Geometry check sheet. Reference: the model listing, model coordinates, mm. Round coordinates to 2 decimals unless told otherwise and drop trailing zeros. Loops run counter-clockwise (first coordinate to the right, second up) from the corner with the lowest first, then second, coordinate; pieces in that order, holes last. Notation, with made-up numbers: M -19.5,66 L 22.5,66 A25 ccw 22.5,81 Z; hole C 23.25,86.25 d1. An arc over 180 degrees is marked long. Write item = value, one per line.
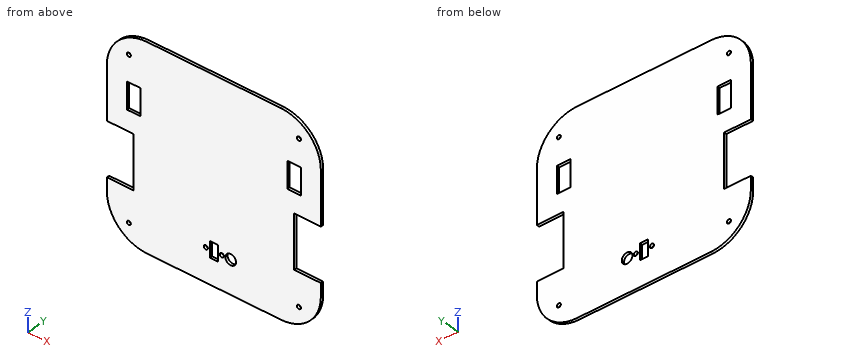
from build123d import *

# Parameters (mm, degrees)
SKETCH1_R           = 1.5
BOSS_EXTRUDE1_DEPTH = 2
SKETCH2_R           = 1.55
SKETCH2_R_2         = 4
SKETCH2_W           = 6
SKETCH2_H           = 12
CUT_EXTRUDE1_DEPTH  = 10
SKETCH3_W           = 10
SKETCH3_H           = 20
CUT_EXTRUDE2_DEPTH  = 10


with BuildPart() as part:
    # Sketch1 → Boss-Extrude1 (new body)
    with BuildSketch(Plane(origin=(0, 0, 0), x_dir=(1, 0, 0), z_dir=(0, 1, 0))):
        with BuildLine():
            Line((-80, 35), (-60, 35))
            Line((-60, 35), (-60, -5))
            Line((-60, -5), (-80, -5))
            Line((-80, -5), (-80, -45))
            ThreePointArc((-80, -45), (-71.213203436, -66.213203436), (-50, -75))
            Line((-50, -75), (50, -75))
            ThreePointArc((50, -75), (71.213203436, -66.213203436), (80, -45))
            Line((80, -45), (80, -5))
            Line((80, -5), (60, -5))
            Line((60, -5), (60, 35))
            Line((60, 35), (80, 35))
            Line((80, 35), (80, 45))
            ThreePointArc((80, 45), (71.213203436, 66.213203436), (50, 75))
            Line((50, 75), (-50, 75))
            ThreePointArc((-50, 75), (-71.213203436, 66.213203436), (-80, 45))
            Line((-80, 45), (-80, 35))
        make_face()
        with Locations(Location((-63.621027185, 59.644712986, 0), (0, 0, 270))):
            Circle(SKETCH1_R, mode=Mode.SUBTRACT)
        with Locations(Location((63.621027185, 59.644712986, 0), (0, 0, 90))):
            Circle(SKETCH1_R, mode=Mode.SUBTRACT)
        with Locations(Location((63.621027185, -59.644712986, 0), (0, 0, 270))):
            Circle(SKETCH1_R, mode=Mode.SUBTRACT)
        with Locations(Location((-63.621027185, -59.644712986, 0), (0, 0, 90))):
            Circle(SKETCH1_R, mode=Mode.SUBTRACT)
    extrude(amount=BOSS_EXTRUDE1_DEPTH)

    # Sketch2 → Cut-Extrude1 (cut)
    with BuildSketch(Plane(origin=(0, 2, 0), x_dir=(1, 0, 0), z_dir=(0, 1, 0))):
        with Locations(Location((-6, 50, 0), (0, 0, 270))):
            Circle(SKETCH2_R)
        with Locations(Location((6, 50, 0), (0, 0, 270))):
            Circle(SKETCH2_R)
        with Locations(Location((12.55, 50, 0), (0, 0, 270))):
            Circle(SKETCH2_R_2)
        with Locations((0, 50)):
            Rectangle(SKETCH2_W, SKETCH2_H)
    extrude(amount=-CUT_EXTRUDE1_DEPTH, mode=Mode.SUBTRACT)

    # Sketch3 → Cut-Extrude2 (cut)
    with BuildSketch(Plane(origin=(0, 2, 0), x_dir=(1, 0, 0), z_dir=(0, 1, 0))):
        with Locations((-60, -30)):
            Rectangle(SKETCH3_W, SKETCH3_H)
        with Locations((60, -30)):
            Rectangle(SKETCH3_W, SKETCH3_H)
    extrude(amount=-CUT_EXTRUDE2_DEPTH, mode=Mode.SUBTRACT)


solid = part.part
(1) Sectioned sample at B-B on z = 2.5. Record the cut outline in (x, y), then the cut area to 3 significant figures.
Result set:
outline = M -60,0 L 60,0 L 60,2 L -60,2 Z
area = 240 mm2
(2) Material ranges on line 1 along Z through (x, y) = (-61, 0.2); line 2 along X through (y, z) = (0.55, -21.5); line 3 along Z through (x, y) = (64.5, 0.9), recorded low to high. Write a range as from..to.
Result set:
line_1 = -72.91..-35, 5..20, 40..72.91
line_2 = -60..60
line_3 = -71.26..-60.86, -58.43..-35, 5..20, 40..58.43, 60.86..71.26
(3) Sectioned sample at C-C on y = 0.4. State how many separate pieces and enclosed holes the cut face has, then the cut area to 3 significant figures.
Result set:
separate_pieces = 1
enclosed_holes = 10
area = 21,100 mm2
(4) Depth check by flat-ended pin: pin 1 Ø3.5 at (x, z) = (63.62, -59.64) entering from -Y; pin 2 Ø0.6 at (x, y) = (58.5, 1) entering from -Z; pin 3 Ø2.5 at (x, z) = (-63.62, 59.64) entering from +Y. Enter the tip coordinate at first touch or a pass-through.
Result set:
pin_1 = 0
pin_2 = -73.86
pin_3 = through
(5) Sectioned sample at A-A on x = 12.55. Record the cut outline in (y, z), then the cut area to 3 significant figures.
Result set:
outline = M 0,-75 L 2,-75 L 2,-54 L 0,-54 Z; M 0,-46 L 2,-46 L 2,75 L 0,75 Z
area = 284 mm2
